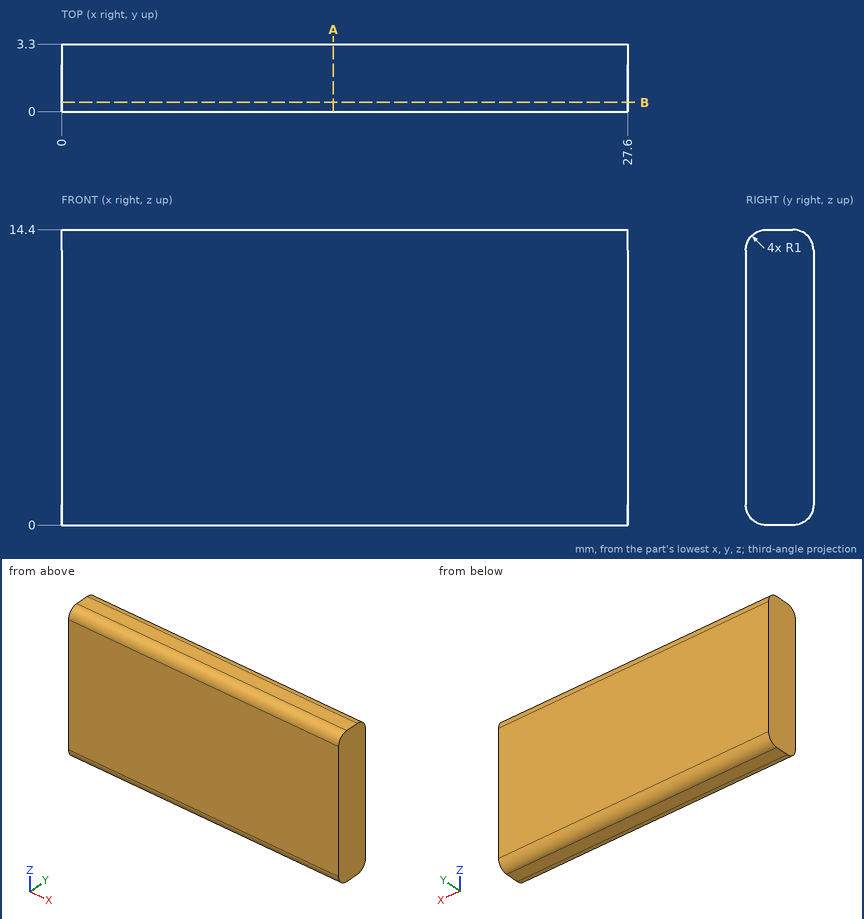
Answer from the drawing. Dimensions are ordinates in mm from the lowest x, y and z of the part. Round coordinates to 2 decimals unless told otherwise and drop trailing zeros. Loops run counter-clockwise (first coordinate to the right, second up) from the corner with the lowest first, then second, coordinate; pieces in that order, holes last.
(1) Find the intervals of material crossed by L1, parallel to Z at x = 11.5, y = 2.4; L2, parallel to Z at x = 23.75, y = 0.2, in increasing order.
Computed values:
L1: z = 0.01 to 14.39
L2: z = 0.4 to 14
(2) The part is cut by section A-A, the plane x = 13.25. Give the vertices of the cut face in (y, z).
Computed values:
outline: (0, 1) arc R1 ccw to (1, 0) - (2.3, 0) arc R1 ccw to (3.3, 1) - (3.3, 13.4) arc R1 ccw to (2.3, 14.4) - (1, 14.4) arc R1 ccw to (0, 13.4) - close
(3) The part is cut by section B-B, the plane y = 0.45. Give the vertices of the cut face in (x, z), and give its area (3 significant figures).
Computed values:
outline: (0, 0.16) - (27.6, 0.16) - (27.6, 14.24) - (0, 14.24) - close
area: 388 mm2
